Design review of the part built by this model. Coordinates are the model's own, in mm. A direction names the side the tool comes from. Give positions to 0.01 mm unless a question says otherwise; leave off trailing zeros. Order: outer loops, then holes, each group sorted by start corner. A loop starts at its lowest first (then second) coordinate and runs counter-clockwise, first axis right, second up. Notation, with made-up numbers: M 48,-39 L 90,-39 A35 ccw 90,-2 Z; hole C -22.75,6 d4. An arc over 180 degrees is marked long. Answer as a JSON object with one key per item and string values.
Autodesk Inventor part; units mm, degrees
ref_plane "Work Plane1" through (0, 43, 0) normal (0, 1, 0) x (-1, 0, 0)
ref_plane "Work Plane3" through (5.1564, 47, -4.5) normal (-0.9999978, 0, 0.0020944) x (0.0020944, 0, 0.9999978)
ref_plane "Work Plane2" through (0.59, 0, 0) normal (1, 0, 0) x (0, 1, 0)
sketch "Sketch1" plane through (0, 0, 0) normal (0, 1, 0) x (-1, 0, 0)
  circle A0 centre (0, 0) radius 4.75
  dimension "d0" = 9.5
  dimension "d31" = 0
ref_plane "Work Plane1" through (0, 43, 0) normal (0, 1, 0) x (-1, 0, 0)
sketch "Sketch2" plane through (0, 43, 0) normal (0, 1, 0) x (-1, 0, 0)
  circle A0 centre (0, 0) radius 3.25
  dimension "d2" = 6.5
  dimension "d32" = 0
loft "Loft1" add profiles "Sketch1", "Sketch2"
sketch "Sketch3" plane through (0, 0, 0) normal (0, -1, 0) x (1, 0, 0)
  circle A0 centre (0, 0) radius 4.75
  line L0 (0, 0) -> (5, 0)
  line L1 (5, 0) -> (5, -10)
  line L2 (5, -10) -> (-5, -10)
  line L3 (-5, -10) -> (-5, 10)
  line L4 (-5, 10) -> (5, 10)
  line L5 (5, 10) -> (5, 0)
  dimension "d7" = 5
  dimension "d8" = 10
  dimension "d9" = 10
  dimension "d10" = 20
  dimension "d11" = 10
  dimension "d33" = 9.5
  dimension "d34" = 5
  dimension "d35" = 0
  dimension "d36" = 5
  dimension "d37" = 0
extrude "Extrusion1" add sketch "Sketch3" along normal blind 3
sketch "Sketch4" plane through (0, 0, 0) normal (0, -1, 0) x (1, 0, 0)
  circle A0 centre (0, 0) radius 5
  dimension "d14" = 10
  dimension "d38" = 0
extrude "Extrusion2" add sketch "Sketch4" along normal blind 3
sketch "Sketch5" plane through (0, 0, 0) normal (0, 1, 0) x (1, 0, 0)
  line L0 (-5, -10) -> (5, -10)
  line L1 (0, -10) -> (0, -7)
  line L2 (0, -7) -> (0, 7)
  circle A0 centre (0, -7) radius 1.5
  circle A1 centre (0, 7) radius 1.5
  point P0 (0, 0)
  point P1 (0, 0)
  dimension "d17" = 3
  dimension "d18" = 14
  dimension "d19" = 3
  dimension "d20" = 3
  dimension "d39" = 0
  dimension "d40" = 10
  dimension "d41" = 5
  dimension "d42" = 0
  dimension "d43" = 10
extrude "Extrusion3" cut sketch "Sketch5" against normal through all
fillet "Fillet1" radius 3 1 edges at (4.75, 0, 0)
sketch "Sketch7" plane through (0, 43, 0) normal (0, 1, 0) x (1, 0, 0)
  line L0 (0, 0) -> (5, 0) construction
  line L1 (5, 0) -> (-5, 0) construction
  line L2 (-5, 0) -> (-5, -9) construction
  line L3 (9, 4.5) -> (-9, 4.5)
  line L4 (-9, 4.5) -> (-9, -5.5)
  line L5 (9, 4.5) -> (9, -5.5)
  line L6 (9, -5.5) -> (-9, -5.5)
  point P0 (-5, 9)
  dimension "d79" = 10
  dimension "d80" = 4.5
  dimension "d81" = 10
  dimension "d82" = 14
  dimension "d83" = 18
  dimension "d84" = 9
  dimension "d85" = 4
  dimension "d86" = 9
  dimension "d87" = 9
extrude "Extrusion5" add sketch "Sketch7" along normal blind 4
fillet "Fillet4" radius 5 1 edges at (3.25, 43, 0)
sketch "Sketch10" plane through (0, 47, 0) normal (0, 1, 0) x (1, 0, 0)
  line L0 (9, -5.5) -> (9, 4.5)
  line L1 (9, -5.5) -> (6.9294, -5.5)
  line L2 (-9, 4.5) -> (-9, 4.5)
  line L3 (-9, 4.5) -> (-9, -5.5)
  line L4 (-9, -5.5) -> (-9, -5.5)
  line L5 (-5.054, 4.5) -> (-5.054, -5.5)
  line L6 (5, 10) -> (5, -10)
  line L7 (5, 4.5) -> (5, -5.5)
  line L8 (-9, 4.5) -> (-5.054, 4.5)
  line L9 (-9, -5.5) -> (-5.054, -5.5)
  line L10 (5, -5.5) -> (9, -5.5)
  line L11 (9, -5.5) -> (9, 4.5)
  line L12 (9, 4.5) -> (9, -5.5)
  line L13 (-9, -5.5) -> (9, -5.5)
  line L14 (5, -5.5) -> (9, -5.5)
  line L15 (9, -5.5) -> (9, 4.5)
  line L16 (5, 4.5) -> (5, -5.5)
  line L17 (9, -5.5) -> (5, -5.5)
  line L18 (9, 4.5) -> (5, 4.5)
  point P0 (0, 0)
  dimension "d102" = 10.054
  dimension "d103" = 90
  dimension "d105" = 90
  dimension "d106" = 2.0706
  dimension "d108" = 18
  dimension "d109" = 18
ref_plane "Work Plane3" through (5.1564, 47, -4.5) normal (-0.9999978, 0, 0.0020944) x (0.0020944, 0, 0.9999978)
ref_plane "Work Plane2" through (0.59, 0, 0) normal (1, 0, 0) x (0, 1, 0)
extrude "Extrusion10" add sketch "Sketch10" along normal blind 21
fillet "Fillet6" radius 5 4 edges at (-7.027, 68, 5.5) (-7.027, 68, -4.5) (7, 68, 5.5) (7, 68, -4.5)
sketch "Sketch12" plane through (9, 43, 5.5) normal (1, 0, 0) x (0, 0, -1)
  arc A0 (10, 20) -> (0, 20) centre (5, 20) ccw
  circle A1 centre (5, 20) radius 3
  point P0 (5.5, -43)
  dimension "d113" = 6
extrude "Extrusion11" cut sketch "Sketch12" against normal blind 21
properties part number "reverse gear crank rod 1"
(1) Draft analysis for pull direction Z (two halves, no side actions). For faces 6 (the cylindrical face through (-7, 66.57, 4)), 7 (the flat face through (-8.6, 43, 0.4)), 8 (the cylindrical face through (-0.325, -1.454, -5.536)), state which applies: +Z half, -Z half, draft (parallel to the pull), parting line (faces both ways), or undercut.
Checked values:
{"face 6": "+Z half", "face 7": "draft", "face 8": "undercut"}
(2) We need section B-B (x = 0). Write out the cut boundary in (y, z).
Checked values:
{"outline": "M -3,-10 L 0,-10 L 0,-8.5 L -3,-8.5 Z; M -3,-5.5 L 0.9,-5.5 A3 cw 2.9,-4.65 L 37.83,-3.43 A5 cw 41.09,-4.5 L 47,-4.5 L 47,5.5 L 42.05,5.5 A5 cw 37.83,3.43 L 2.9,4.65 A3 cw 0.9,5.5 L -3,5.5 Z; M -3,8.5 L 0,8.5 L 0,10 L -3,10 Z"}
(3) Tool access review of faces 1 (the flat face through (-5, -1, 0)), 2 (the flat face through (5, -1, 0)), 3 (the flat face through (0, -1, -10)), 4 (the conical face through (0.88, 20.12, 3.95)), 5 (the flat face through (0, 47, 0)): name each direction out of +Z, -Z, +X, -X, +Y, -Y from which nothing blocks a thin tool from reaching the whole face with its end or side.
Checked values:
{"face 1": "+Z, -Z, -X, -Y", "face 2": "+Z, -Z, +X, -Y", "face 3": "-Z, +X, -X, +Y, -Y", "face 4": "none", "face 5": "+Z, -Z, +Y"}
(4) We need section C-C (y = 13.5). Write out the cut boundary in (x, z).
Checked values:
{"outline": "C 0,0 d8.56"}
(5) We need section A-A (y = 58). Write out the cut boundary in (x, z), plus the area to 3 significant figures.
Checked values:
{"outline": "M -9,-4.5 L -5.05,-4.5 L -5.05,5.5 L -9,5.5 Z; M 5,-4.5 L 9,-4.5 L 9,5.5 L 5,5.5 Z", "area": "79.5 mm^2"}
(6) To check wall thickness, follow L1, parallel to Z at x = 0, y = -0.1; L2, parallel to X at y = 57, z = -1; L3, parallel to X at y = -1.4, z = 7. State the ranges of each line that lie inside material, in increasing order. Write a range as from..to.
Checked values:
{"L1": "z = -10..-8.5, -5.5..5.5, 8.5..10", "L2": "x = -9..-5.05, 5..9", "L3": "x = -5..-1.5, 1.5..5"}
(7) Insertion check: pin 1 (3.5 mm diameter, centred on x = 0, z = -7, fed in from +Y); pin 2 (3.5 mm diameter, centred on x = 0.5, z = -8.5, fed in from +Y); pin 3 (4 mm diameter, centred on x = 0, z = 7, fed in from +Y). Each pin has a flat end and moves straight along its axis. Give the tip position at first contact, or say it passes through.
Checked values:
{"pin 1": "stops at y = 1.2", "pin 2": "stops at y = 0.03", "pin 3": "stops at y = 47"}
